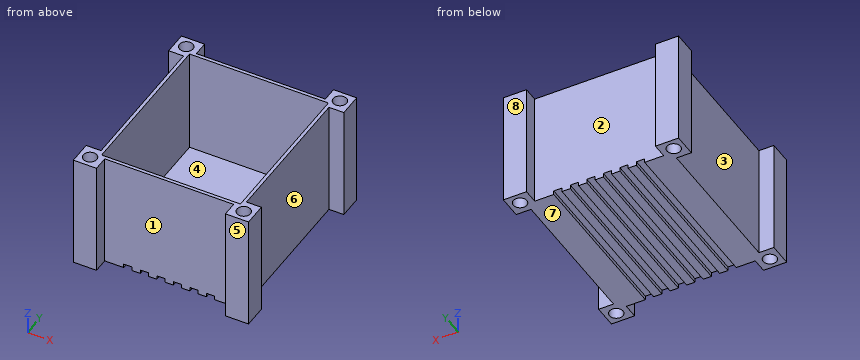
```python
from build123d import *

# Parameters (mm, degrees)
F0_W     = 2.5
F0_H     = 2.5
F1_DEPTH = 35
F2_R     = 2.05
F3_DEPTH = 35
F4_W     = 42
F4_H     = 48
F5_DEPTH = 32
F6_W     = 2.5
F6_H     = 1.2
F7_DEPTH = 50


with BuildPart() as f1:
    # F0 (on Top) → F1 (new body)
    with BuildSketch(Plane.XY):
        Polygon((-22, 22.5), (-22, 25), (-19.5, 25), (-19.5, 29.5), (-26.5, 29.5), (-26.5, 22.5), align=None)
        with Locations((-20.75, 23.75)):
            Rectangle(F0_W, F0_H)
        Polygon((19.5, 25), (-19.5, 25), (-19.5, 22.5), (-22, 22.5), (-22, -22.5), (-19.5, -22.5), (-19.5, -25), (19.5, -25), (19.5, -22.5), (22, -22.5), (22, 22.5), (19.5, 22.5), align=None)
        Polygon((19.5, 29.5), (19.5, 25), (22, 25), (22, 22.5), (26.5, 22.5), (26.5, 29.5), align=None)
        with Locations((20.75, 23.75)):
            Rectangle(F0_W, F0_H)
        with Locations((-20.75, -23.75)):
            Rectangle(F0_W, F0_H)
        Polygon((-22, -25), (-22, -22.5), (-26.5, -22.5), (-26.5, -29.5), (-19.5, -29.5), (-19.5, -25), align=None)
        Polygon((26.5, -22.5), (22, -22.5), (22, -25), (19.5, -25), (19.5, -29.5), (26.5, -29.5), align=None)
        with Locations((20.75, -23.75)):
            Rectangle(F0_W, F0_H)
    extrude(amount=F1_DEPTH)

    # F2 (on face) → F3 (cut, through all)
    with BuildSketch(Plane.XY.offset(35)):
        with Locations((-23.25, 26.25)):
            Circle(F2_R)
        with Locations((23.25, 26.25)):
            Circle(F2_R)
        with Locations((-23.25, -26.25)):
            Circle(F2_R)
        with Locations((23.25, -26.25)):
            Circle(F2_R)
    extrude(amount=-F3_DEPTH, mode=Mode.SUBTRACT)

    # F4 (on face) → F5 (cut)
    with BuildSketch(Plane.XY.offset(35)):
        Rectangle(F4_W, F4_H)
    extrude(amount=-F5_DEPTH, mode=Mode.SUBTRACT)

    # F6 (on face) → F7 (cut, through all)
    with BuildSketch(Plane(origin=(0, 25, 0), x_dir=(-1, 0, 0), z_dir=(0, 1, 0))):
        with Locations((12.5, 0.6)):
            Rectangle(F6_W, F6_H)
        with Locations((7.5, 0.6)):
            Rectangle(F6_W, F6_H)
        with Locations((2.5, 0.6)):
            Rectangle(F6_W, F6_H)
        with Locations((-2.5, 0.6)):
            Rectangle(F6_W, F6_H)
        with Locations((-7.5, 0.6)):
            Rectangle(F6_W, F6_H)
        with Locations((-12.5, 0.6)):
            Rectangle(F6_W, F6_H)
    extrude(amount=-F7_DEPTH, mode=Mode.SUBTRACT)


solid = f1.part
```
Geometry: final body of the model. Coordinates: model frame, mm. Face numbers are marked on the shaded views. A direction names the side the tool comes from. Give positions to 0.01 mm unless a question says otherwise; leave off trailing zeros. Loops run counter-clockwise (first coordinate to the right, second up) from the corner with the lowest first, then second, coordinate; pieces in that order, holes last. Notation, with made-up numbers: (65.25, 87) - (74.25, 87) arc R7 cw to (74.25, 92) - close; hole circle Ø9 at (-16, -4.75). An arc over 180 degrees is marked (long way). Answer as CSV lines item,"result". Start each with the question number.
(1) Section query B-B (x = 23.25). Output: boundary loops of the cut face in (y, z), and give its area (3 significant figures).
(2) Pin query (flat end, axial travel): P1, Ø1, axis at y = 9.5, z = 1, coming from the +X side; P2, Ø1, axis at y = -12, z = 0.5, coming from the -X side; P3, Ø8, axis at x = -12, z = 6.5, coming from the +Y side; P4, Ø2.5, axis at x = 23.25, y = 26.25, coming from the +Z side. Return the tip coordinate at first contact, or that it passes through.
(3) Section query D-D (x = 8). Output: boundary loops of the cut face in (y, z), and give its area (3 significant figures).
(4) Mould query, pull axis Y, two halves, no side actions, for the marked faces 6, 7 and 8. Classes: +Y half, -Y half, draft (parallel to the pull), parting line (faces both ways), or undercut.
(5) Reachability of the marked faces 1, 2, 3, 4 and 5 from +Z, -Z, +X, -X, +Y, -Y: full face, straight path, thin tool, end or side. Return the list, or none.
(6) Section query A-A (z = 12). Output: boundary loops of the cut face in (x, y).
(7) Ray query, line 1 along Y through (x, z) = (-23.25, 26); line 2 along Y through (x, z) = (15, 25.5); line 3 along X through (y, z) = (16, 17.5). Return the intervals inside material, ascending. Write a range as [from, to].
(8) Section query C-C (y = -26.25). Output: boundary loops of the cut face in (x, z).
Worked answers:
1,outline,"(-29.5, 0) - (-28.3, 0) - (-28.3, 35) - (-29.5, 35) - close; (-24.2, 0) - (-22.5, 0) - (-22.5, 35) - (-24.2, 35) - close; (22.5, 0) - (24.2, 0) - (24.2, 35) - (22.5, 35) - close; (28.3, 0) - (29.5, 0) - (29.5, 35) - (28.3, 35) - close"
1,area,"203 mm^2"
2,P1,"stops at x = 22"
2,P2,"stops at x = -22"
2,P3,"stops at y = 25"
2,P4,"passes through"
3,outline,"(-25, 1.2) - (25, 1.2) - (25, 35) - (24, 35) - (24, 3) - (-24, 3) - (-24, 35) - (-25, 35) - close"
3,area,"154 mm^2"
4,face 6,"undercut"
4,face 7,"draft"
4,face 8,"+Y half"
5,face 1,"+Z, -Z, -Y"
5,face 2,"+Z, -Z, +Y"
5,face 3,"+Z, -Z, -X"
5,face 4,"+Z"
5,face 5,"+Z, -Z, +X, -X, -Y"
6,outline,"(-26.5, -29.5) - (-19.5, -29.5) - (-19.5, -25) - (19.5, -25) - (19.5, -29.5) - (26.5, -29.5) - (26.5, -22.5) - (22, -22.5) - (22, 22.5) - (26.5, 22.5) - (26.5, 29.5) - (19.5, 29.5) - (19.5, 25) - (-19.5, 25) - (-19.5, 29.5) - (-26.5, 29.5) - (-26.5, 22.5) - (-22, 22.5) - (-22, -22.5) - (-26.5, -22.5) - close; hole circle Ø4.1 at (-23.25, -26.25); hole circle Ø4.1 at (-23.25, 26.25); hole (-21, -24) - (21, -24) - (21, 24) - (-21, 24) - close; hole circle Ø4.1 at (23.25, -26.25); hole circle Ø4.1 at (23.25, 26.25)"
7,line 1,"y = [-29.5, -28.3], [-24.2, -22.5], [22.5, 24.2], [28.3, 29.5]"
7,line 2,"y = [-25, -24], [24, 25]"
7,line 3,"x = [-22, -21], [21, 22]"
8,outline,"(-26.5, 0) - (-25.3, 0) - (-25.3, 35) - (-26.5, 35) - close; (-21.2, 0) - (-19.5, 0) - (-19.5, 35) - (-21.2, 35) - close; (19.5, 0) - (21.2, 0) - (21.2, 35) - (19.5, 35) - close; (25.3, 0) - (26.5, 0) - (26.5, 35) - (25.3, 35) - close"
